The listing builds one solid part. Answer for the finished solid, in the listing's coordinates (mm). A direction names the side the tool comes from. Coordinates: 2 decimals unless noted, no trailing zeros. Write each loop counter-clockwise with the first axis right and the second up, starting at its lowest first coordinate (ties: lowest second). Pieces come first, ordered by that corner, then holes. Notation, with made-up numbers: M -26.75,58 L 20.25,58 A17 cw 20.25,71 Z; hole C 70.5,-5 d1. An arc over 180 degrees is marked long. Answer as CSV lines item,"result".
```python
from build123d import *

# Parameters (mm, degrees)
SKETCH2_R           = 1.15
RESISTOR_BODY_DEPTH = 5.6
LEAD1_PROFILE_R     = 0.275
SKETCH6_R           = 0.275
LEAD2_DEPTH         = 9.4


with BuildPart() as part:
    # Sketch2 → Resistor Body (new body)
    with BuildSketch(Plane.XY):
        Circle(SKETCH2_R)
    extrude(amount=RESISTOR_BODY_DEPTH)

    # Lead1: sweep along a path in Lead1 Path
    with BuildLine(Plane(origin=(0, 0, 0), x_dir=(1, 0, 0), z_dir=(0, 1, 0))) as lead1_path:
        Line((0, -5.6), (0, -7.6))
        ThreePointArc((0, -7.6), (0.585786438, -9.014213562), (2, -9.6))
        Line((2, -9.6), (3, -9.6))
        ThreePointArc((3, -9.6), (4.414213562, -9.014213562), (5, -7.6))
        Line((5, -7.6), (5, 9.4))
    # Lead1 Profile → Lead1 (sweep)
    with BuildSketch(Plane(origin=(0, 0, 5.6), x_dir=(-1, 0, 0), z_dir=(0, 0, 1))):
        Circle(LEAD1_PROFILE_R)
    sweep(path=lead1_path.line)

    # Sketch6 → Lead2 (add)
    with BuildSketch(Plane(origin=(0, 0, 0), x_dir=(1, 0, 0), z_dir=(0, 0, -1))):
        Circle(SKETCH6_R)
    extrude(amount=LEAD2_DEPTH)


solid = part.part
```
Q1. Find section B-B (z = 1.75). Give the vertices of the cut face in (x, y) (3 decimals).
Output:
outline,"C 0,0 d2.3; C 5,0 d0.55"
Q2. For faces 1 (the flat face through (0, -0.5, 0)), 2 (the flat face through (0, -0.5, 5.6)), determine the directions among +Z, -Z, +X, -X, +Y, -Y from which every point of the face is accessible in a straight line to the end or side of a thin tool.
Output:
face 1,"-Z"
face 2,"none"
Q3. Find section D-D (x = -0.5). Give the vertices of the cut face in (y, z).
Output:
outline,"M -1.04,0 L 1.04,0 L 1.04,5.6 L -1.04,5.6 Z"
Q4. Flat-ended cylindrical pins translate along their axes: pin 1 Ø1 at (x, y) = (1, 0.5) entering from +Z; pin 2 Ø1 at (y, z) = (-0.5, -1.5) entering from -X (3 decimals); pin 3 Ø1 at (x, z) = (3, -3.5) entering from +Y. Find the tip coordinate at first contact, or state that the pin passes through.
Output:
pin 1,"z = 9.74"
pin 2,"x = -0.275"
pin 3,"through"
Q5. Straight lines are drawn through the part: line 1 (X direction, y = 0.05, z = -0.25); line 2 (X direction, y = 0.2, z = -3.75); line 3 (Z direction, x = 3.5, y = 0.05). For each, find the intervals that lie inside material, in ascending order.
Output:
line 1,"-0.27 to 0.27, 4.73 to 5.27"
line 2,"-0.19 to 0.19, 4.81 to 5.19"
line 3,"9.26 to 9.81"
Q6. Find section C-C (z = 7). Give the vertices of the cut face in (x, y) (3 decimals), and give its area (3 significant figures).
Output:
outline,"C 0,0 d0.55; C 5,0 d0.55"
area,"0.475 mm2"
Q7. Find section A-A (y = 0). Give the vertices of the cut face in (x, z) (3 decimals).
Output:
outline,"M -1.15,0 L -0.275,0 L -0.275,-9.4 L 0.275,-9.4 L 0.275,0 L 1.15,0 L 1.15,5.6 L 0.275,5.6 L 0.275,7.6 A1.725 cw 2,9.325 L 3,9.325 A1.725 cw 4.725,7.6 L 4.725,-9.4 L 5.275,-9.4 L 5.275,7.6 A2.275 ccw 3,9.875 L 2,9.875 A2.275 ccw -0.275,7.6 L -0.275,5.6 L -1.15,5.6 Z"
